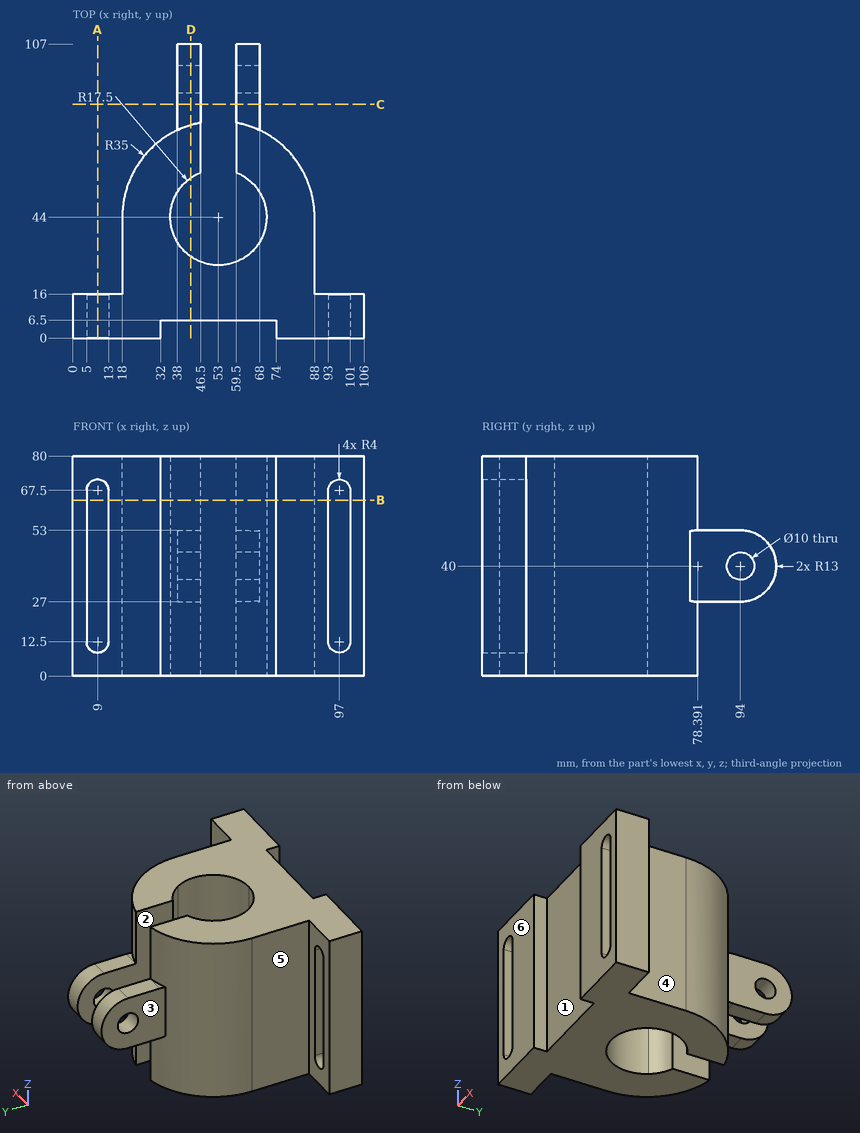
Print and shaded views of the part. All mm, measured from the part's lowest x, y and z. A direction names the side the tool comes from. Give positions to 0.01 mm unless a question says otherwise; leave off trailing zeros. Order: outer loops, then holes, each group sorted by start corner. A loop starts at its lowest first (then second) coordinate and runs counter-clockwise, first axis right, second up. Notation, with made-up numbers: M 88,-37.75 L 134,-37.75 A13 cw 134,-12.75 Z; hole C -21,33.25 d5. An arc over 180 degrees is marked long. Use one line per item in the form item = value.
Q1. Slice it at D-D, the plane x = 43. Write the cut outline in (y, z).
Conclusion:
outline = M 6.5,0 L 29.64,0 L 29.64,80 L 6.5,80 Z; M 58.36,0 L 77.54,0 L 77.54,27.03 A13 ccw 78.39,27 L 94,27 A13 ccw 94,53 L 78.39,53 A13 ccw 77.54,52.97 L 77.54,80 L 58.36,80 Z; hole C 94,40 d10
Q2. Slice it at B-B, the plane z = 64. Write the cut outline in (x, y).
Conclusion:
outline = M 0,0 L 5,0 L 5,16 L 0,16 Z; M 13,0 L 32,0 L 32,6.5 L 74,6.5 L 74,0 L 93,0 L 93,16 L 88,16 L 88,44 A35 ccw 59.5,78.39 L 59.5,60.25 A17.5 cw long 46.5,60.25 L 46.5,78.39 A35 ccw 18,44 L 18,16 L 13,16 Z; M 101,0 L 106,0 L 106,16 L 101,16 Z
Q3. Slice it at A-A, the plane x = 9. Write the cut outline in (y, z), and give its area (3 significant figures).
Conclusion:
outline = M 0,0 L 16,0 L 16,8.5 L 0,8.5 Z; M 0,71.5 L 16,71.5 L 16,80 L 0,80 Z
area = 272 mm2
Q4. Slice it at C-C, the plane y = 85. Write the cut outline in (x, z), and give its area (3 significant figures).
Conclusion:
outline = M 38,27 L 46.5,27 L 46.5,53 L 38,53 Z; M 59.5,27 L 68,27 L 68,53 L 59.5,53 Z
area = 442 mm2
Q5. Which spindle directions (+Z, -Z, +X, -X, +Y, -Y) get a long thin tool onto all of the face, cutting with end or side? Do the marked faces 1, 2, 3 and 4. Say none if no direction does.
Conclusion:
face_1 = +Z, -Z, -Y
face_2 = +Z, -Z, +Y
face_3 = +Z, -Z, -X, +Y
face_4 = +Z, -Z, +X, +Y
Q6. Wall check: probe 1 along Z at (x, y) = (40, 94); probe 2 along X at (y, z) = (79.5, 28); probe 3 along Y at (x, z) = (15, 21.5). Give the ranges that are in metal, low to high.
Conclusion:
probe_1 = 27 to 35, 45 to 53
probe_2 = 38 to 46.5, 59.5 to 68
probe_3 = 0 to 16
Q7. Pin check, flat tips, straight feed: P1, Ø8.5, axis at y = 33, z = 37, coming from the +X side; P2, Ø2, axis at x = 66, z = 68, coming from the -Y side; P3, Ø4, axis at x = 42, y = 84.5, coming from the -Z side; P4, Ø8, axis at y = 94, z = 40, coming from the -X side. Stop position of each tip, or through.
Conclusion:
P1 = 88
P2 = 6.5
P3 = 27
P4 = through
Q8. Pull direction Y, two halves, no side cores. Call the marked faces 5 and 6: released by +Y, released by -Y, zero draft, split by the parting line, or undercut.
Conclusion:
face_5 = zero draft
face_6 = released by -Y
